```python
from build123d import *

# Parameters (mm, degrees)
EXTRUDE_1_DEPTH     = 9.4
CUT_EXTRUDE_1_DEPTH = 7.8
EXTRUDE_2_DEPTH     = 3.8
CUT_EXTRUDE_2_DEPTH = 1.8
SKETCH_5_R          = 1
CUT_EXTRUDE_4_DEPTH = 3.8
CUT_EXTRUDE_5_DEPTH = 2.8
CUT_EXTRUDE_6_DEPTH = 2.8
CUT_EXTRUDE_7_DEPTH = 2.8
EXTRUDE_3_DEPTH     = 1.6
CUT_EXTRUDE_8_DEPTH = 3.2


with BuildPart() as part:
    # 草图1 → 凸台-拉伸1 (new body)
    with BuildSketch(Plane(origin=(0, 0, 0), x_dir=(1, 0, 0), z_dir=(0, 1, 0))):
        with BuildLine():
            Line((-22.3, -22.35), (22.3, -22.35))
            ThreePointArc((22.3, -22.35), (23.714213562, -21.764213562), (24.3, -20.35))
            Line((24.3, -20.35), (24.3, 20.35))
            ThreePointArc((24.3, 20.35), (23.714213562, 21.764213562), (22.3, 22.35))
            Line((22.3, 22.35), (-22.3, 22.35))
            ThreePointArc((-22.3, 22.35), (-23.714213562, 21.764213562), (-24.3, 20.35))
            Line((-24.3, 20.35), (-24.3, -20.35))
            ThreePointArc((-24.3, -20.35), (-23.714213562, -21.764213562), (-22.3, -22.35))
        make_face()
    extrude(amount=EXTRUDE_1_DEPTH)

    # 草图2 → 切除-拉伸1 (cut)
    with BuildSketch(Plane(origin=(0, 9.4, 0), x_dir=(1, 0, 0), z_dir=(0, 1, 0))):
        with BuildLine():
            Line((-20.7, -20.75), (20.7, -20.75))
            ThreePointArc((20.7, -20.75), (22.114213562, -20.164213562), (22.7, -18.75))
            Line((22.7, -18.75), (22.7, 18.75))
            ThreePointArc((22.7, 18.75), (22.114213562, 20.164213562), (20.7, 20.75))
            Line((20.7, 20.75), (-20.7, 20.75))
            ThreePointArc((-20.7, 20.75), (-22.114213562, 20.164213562), (-22.7, 18.75))
            Line((-22.7, 18.75), (-22.7, -18.75))
            ThreePointArc((-22.7, -18.75), (-22.114213562, -20.164213562), (-20.7, -20.75))
        make_face()
    extrude(amount=-CUT_EXTRUDE_1_DEPTH, mode=Mode.SUBTRACT)

    # 草图3 → 凸台-拉伸2 (add)
    with BuildSketch(Plane(origin=(0, 1.6, 0), x_dir=(1, 0, 0), z_dir=(0, 1, 0))):
        with BuildLine():
            Line((-21.2, -14.15), (-17.6, -14.15))
            ThreePointArc((-17.6, -14.15), (-16.539339828, -14.589339828), (-16.1, -15.65))
            Line((-16.1, -15.65), (-16.1, -19.25))
            ThreePointArc((-16.1, -19.25), (-16.539339828, -20.310660172), (-17.6, -20.75))
            Line((-17.6, -20.75), (-22.7, -20.75))
            Line((-22.7, -20.75), (-22.7, -15.65))
            ThreePointArc((-22.7, -15.65), (-22.260660172, -14.589339828), (-21.2, -14.15))
        make_face()
        with BuildLine():
            Line((-22.7, 20.75), (-17.6, 20.75))
            ThreePointArc((-17.6, 20.75), (-16.539339828, 20.310660172), (-16.1, 19.25))
            Line((-16.1, 19.25), (-16.1, 15.65))
            ThreePointArc((-16.1, 15.65), (-16.539339828, 14.589339828), (-17.6, 14.15))
            Line((-17.6, 14.15), (-21.2, 14.15))
            ThreePointArc((-21.2, 14.15), (-22.260660172, 14.589339828), (-22.7, 15.65))
            Line((-22.7, 15.65), (-22.7, 20.75))
        make_face()
        with BuildLine():
            Line((19.7, 15.65), (19.7, 19.25))
            ThreePointArc((19.7, 19.25), (19.260660172, 20.310660172), (18.2, 20.75))
            Line((18.2, 20.75), (14.6, 20.75))
            ThreePointArc((14.6, 20.75), (13.539339828, 20.310660172), (13.1, 19.25))
            Line((13.1, 19.25), (13.1, 15.65))
            ThreePointArc((13.1, 15.65), (13.539339828, 14.589339828), (14.6, 14.15))
            Line((14.6, 14.15), (18.2, 14.15))
            ThreePointArc((18.2, 14.15), (19.260660172, 14.589339828), (19.7, 15.65))
        make_face()
        with BuildLine():
            Line((18.2, -14.15), (14.6, -14.15))
            ThreePointArc((14.6, -14.15), (13.539339828, -14.589339828), (13.1, -15.65))
            Line((13.1, -15.65), (13.1, -19.25))
            ThreePointArc((13.1, -19.25), (13.539339828, -20.310660172), (14.6, -20.75))
            Line((14.6, -20.75), (18.2, -20.75))
            ThreePointArc((18.2, -20.75), (19.260660172, -20.310660172), (19.7, -19.25))
            Line((19.7, -19.25), (19.7, -15.65))
            ThreePointArc((19.7, -15.65), (19.260660172, -14.589339828), (18.2, -14.15))
        make_face()
    extrude(amount=EXTRUDE_2_DEPTH)

    # 草图4 → 切除-拉伸2 (cut)
    with BuildSketch(Plane(origin=(0, 5.4, 0), x_dir=(1, 0, 0), z_dir=(0, 1, 0))):
        Polygon((-18.328981591, -19.607194502), (-17.132908096, -17.564465561), (-18.303926505, -15.507271059), (-20.671018409, -15.492805498), (-21.867091904, -17.535534439), (-20.696073495, -19.592728941), align=None)
        Polygon((-20.696073495, 19.592728941), (-18.328981591, 19.607194502), (-17.132908096, 17.564465561), (-18.303926505, 15.507271059), (-20.671018409, 15.492805498), (-21.867091904, 17.535534439), align=None)
        Polygon((18.867091904, 17.535534439), (17.696073495, 19.592728941), (15.328981591, 19.607194502), (14.132908096, 17.564465561), (15.303926505, 15.507271059), (17.671018409, 15.492805498), align=None)
    extrude(amount=-CUT_EXTRUDE_2_DEPTH, mode=Mode.SUBTRACT)

    # 草图5 → 切除-拉伸4 (cut)
    with BuildSketch(Plane(origin=(0, 5.4, 0), x_dir=(1, 0, 0), z_dir=(0, 1, 0))):
        with Locations(Location((-19.5, -17.55, 0), (0, 0, 270))):
            Circle(SKETCH_5_R)
        with Locations(Location((-19.5, 17.55, 0), (0, 0, 270))):
            Circle(SKETCH_5_R)
        with Locations(Location((16.5, 17.55, 0), (0, 0, 270))):
            Circle(SKETCH_5_R)
    extrude(amount=-CUT_EXTRUDE_4_DEPTH, mode=Mode.SUBTRACT)

    # 草图6 → 切除-拉伸5 (cut)
    with BuildSketch(Plane.ZY.offset(24.3)):
        with BuildLine():
            Line((-13.25, 6.9), (-4.05, 6.9))
            ThreePointArc((-4.05, 6.9), (-3.696446609, 7.046446609), (-3.55, 7.4))
            Line((-3.55, 7.4), (-3.55, 10.4))
            Line((-3.55, 10.4), (-13.75, 10.4))
            Line((-13.75, 10.4), (-13.75, 7.4))
            ThreePointArc((-13.75, 7.4), (-13.603553391, 7.046446609), (-13.25, 6.9))
        make_face()
    extrude(amount=-CUT_EXTRUDE_5_DEPTH, mode=Mode.SUBTRACT)

    # 草图7 → 切除-拉伸6 (cut)
    with BuildSketch(Plane.XY.offset(22.35)):
        with BuildLine():
            Line((-14.7, 8.9), (-9.3, 8.9))
            ThreePointArc((-9.3, 8.9), (-9.087867966, 8.812132034), (-9, 8.6))
            Line((-9, 8.6), (-9, 7.2))
            ThreePointArc((-9, 7.2), (-9.087867966, 6.987867966), (-9.3, 6.9))
            Line((-9.3, 6.9), (-14.7, 6.9))
            ThreePointArc((-14.7, 6.9), (-14.912132034, 6.987867966), (-15, 7.2))
            Line((-15, 7.2), (-15, 8.6))
            ThreePointArc((-15, 8.6), (-14.912132034, 8.812132034), (-14.7, 8.9))
        make_face()
    extrude(amount=-CUT_EXTRUDE_6_DEPTH, mode=Mode.SUBTRACT)

    # 草图8 → 切除-拉伸7 (cut)
    with BuildSketch(Plane.XY.offset(22.35)):
        with BuildLine():
            Line((3.7, 8.1), (7.3, 8.1))
            ThreePointArc((7.3, 8.1), (7.441421356, 8.041421356), (7.5, 7.9))
            Line((7.5, 7.9), (7.5, 7.1))
            ThreePointArc((7.5, 7.1), (7.441421356, 6.958578644), (7.3, 6.9))
            Line((7.3, 6.9), (3.7, 6.9))
            ThreePointArc((3.7, 6.9), (3.558578644, 6.958578644), (3.5, 7.1))
            Line((3.5, 7.1), (3.5, 7.9))
            ThreePointArc((3.5, 7.9), (3.558578644, 8.041421356), (3.7, 8.1))
        make_face()
    extrude(amount=-CUT_EXTRUDE_7_DEPTH, mode=Mode.SUBTRACT)

    # 草图12 → 凸台-拉伸3 (add, symmetric)
    with BuildSketch(Plane(origin=(0, 1.6, 0), x_dir=(1, 0, 0), z_dir=(0, 1, 0))):
        with BuildLine():
            Line((-27.3, 11.5), (-24.3, 11.5))
            Line((-24.3, 11.5), (-24.3, -11.5))
            Line((-24.3, -11.5), (-27.3, -11.5))
            ThreePointArc((-27.3, -11.5), (-28.007106781, -11.207106781), (-28.3, -10.5))
            Line((-28.3, -10.5), (-28.3, 10.5))
            ThreePointArc((-28.3, 10.5), (-28.007106781, 11.207106781), (-27.3, 11.5))
        make_face()
        with BuildLine():
            Line((27.3, -11.5), (24.3, -11.5))
            Line((24.3, -11.5), (24.3, 11.5))
            Line((24.3, 11.5), (27.3, 11.5))
            ThreePointArc((27.3, 11.5), (28.007106781, 11.207106781), (28.3, 10.5))
            Line((28.3, 10.5), (28.3, -10.5))
            ThreePointArc((28.3, -10.5), (28.007106781, -11.207106781), (27.3, -11.5))
        make_face()
    extrude(amount=EXTRUDE_3_DEPTH, both=True)

    # 草图13 → 切除-拉伸8 (cut)
    with BuildSketch(Plane(origin=(0, 3.2, 0), x_dir=(1, 0, 0), z_dir=(0, 1, 0))):
        with BuildLine():
            Line((-25.3, 9.5), (-24.3, 9.5))
            Line((-24.3, 9.5), (-24.3, -9.5))
            Line((-24.3, -9.5), (-25.3, -9.5))
            ThreePointArc((-25.3, -9.5), (-26.007106781, -9.207106781), (-26.3, -8.5))
            Line((-26.3, -8.5), (-26.3, 8.5))
            ThreePointArc((-26.3, 8.5), (-26.007106781, 9.207106781), (-25.3, 9.5))
        make_face()
        with BuildLine():
            Line((25.3, -9.5), (24.3, -9.5))
            Line((24.3, -9.5), (24.3, 9.5))
            Line((24.3, 9.5), (25.3, 9.5))
            ThreePointArc((25.3, 9.5), (26.007106781, 9.207106781), (26.3, 8.5))
            Line((26.3, 8.5), (26.3, -8.5))
            ThreePointArc((26.3, -8.5), (26.007106781, -9.207106781), (25.3, -9.5))
        make_face()
    extrude(amount=-CUT_EXTRUDE_8_DEPTH, mode=Mode.SUBTRACT)


solid = part.part
```
Part model, mm, in its own coordinate system. A direction names the side the tool comes from. Coordinates: 2 decimals unless noted, no trailing zeros. Write each loop counter-clockwise with the first axis right and the second up, starting at its lowest first coordinate (ties: lowest second). Pieces come first, ordered by that corner, then holes.
Item 1: Which spindle directions (+Z, -Z, +X, -X, +Y, -Y) get a long thin tool onto all of the face, cutting with end or side? Do faces 1 (the face through (-24, 6.9, -9)), 2 (the face through (0, 0, 0)), 3 (the face through (6, 6.9, 22)), 4 (the face through (-17.71, 4.51, 16.55)). Say none if no direction does.
Item 2: Slice it at A-A (x = -10). Write the cut outline in (y, z).
Item 3: Mould opens along X. For faces 5 (the face through (-23.7, 4.63, -21.78)), 6 (the face through (0, 5, 22.35)), 7 (the face through (0, 6, 20.75)) say: released by +X, released by -X, zero draft, split by the parting line, or undercut.
Item 4: Pin check, flat tips, straight feed: pin 1 (8 mm diameter, centred on x = 13.5, z = -2, fed in from +Y); pin 2 (2 mm diameter, centred on x = -18.5, z = -16.5, fed in from +Y); pin 3 (0.5 mm diameter, centred on x = -25, y = 1, fed in from -Z). Stop position of each tip, or through.
Item 5: Slice it at B-B (z = 7). Write the cut outline in (x, y).
Item 6: Slice it at C-C (y = 2.25). Count the separate pieces of the cut face and the enclosed holes in it, and give its area (3 significant figures).
Item 7: Probe line 1 (X direction, y = 2.95, z = -17.55); line 2 (X direction, y = 3.1, z = 17.55); line 3 (Z direction, x = -18.5, y = 4). List the from-to ranges inside material, lowest first.
Item 8: Slice it at D-D (z = -6.5). Write the cut outline in (x, y), and give its area (3 significant figures).
Results found:
1. face 1: -X, +Y
1. face 2: +Z, -Z, +X, -X, -Y
1. face 3: +Z
1. face 4: +Y
2. outline: (0, -22.35) - (9.4, -22.35) - (9.4, -20.75) - (1.6, -20.75) - (1.6, 20.75) - (6.9, 20.75) - (6.9, 22.35) - (0, 22.35) - close; (8.9, 20.75) - (9.4, 20.75) - (9.4, 22.35) - (8.9, 22.35) - close
3. face 5: released by -X
3. face 6: zero draft
3. face 7: undercut
4. pin 1: stops at y = 1.6
4. pin 2: stops at y = 5.4
4. pin 3: stops at z = -11.5
5. outline: (-28.3, 0) - (-26.3, 0) - (-26.3, 3.2) - (-28.3, 3.2) - close; (-24.3, 0) - (24.3, 0) - (24.3, 9.4) - (22.7, 9.4) - (22.7, 1.6) - (-22.7, 1.6) - (-22.7, 9.4) - (-24.3, 9.4) - close; (26.3, 0) - (28.3, 0) - (28.3, 3.2) - (26.3, 3.2) - close
6. separate pieces: 1
6. enclosed holes: 6
6. area: 553 mm2
7. line 1: x = -24.3 to -20.5, -18.5 to -16.1, 13.1 to 15.5, 17.5 to 19.7, 22.7 to 24.3
7. line 2: x = -24.3 to -20.5, -18.5 to -16.1, 13.1 to 19.7, 22.7 to 24.3
7. line 3: z = -22.35 to -19.61, -15.51 to -14.15, 14.15 to 15.51, 19.61 to 22.35
8. outline: (-28.3, 0) - (-26.3, 0) - (-26.3, 3.2) - (-28.3, 3.2) - close; (-24.3, 0) - (24.3, 0) - (24.3, 9.4) - (22.7, 9.4) - (22.7, 1.6) - (-22.7, 1.6) - (-22.7, 6.9) - (-24.3, 6.9) - close; (26.3, 0) - (28.3, 0) - (28.3, 3.2) - (26.3, 3.2) - close
8. area: 112 mm2
